```python
from build123d import *

# Parameters (mm, degrees)
SKETCH1_R                  = 15
BOSS_EXTRUDE1_DEPTH        = 210
FILLET1_R                  = 4
CHAMFER1_SIZE              = 1
M8X1_25_TAPPED_HOLE1_D     = 6.8
M8X1_25_TAPPED_HOLE1_DEPTH = 19.75
M8X1_25_TAPPED_HOLE1_TIP   = 2.042926105


with BuildPart() as part:
    # Sketch1 → Boss-Extrude1 (new body)
    with BuildSketch(Plane(origin=(0, 0, 0), x_dir=(1, 0, 0), z_dir=(0, 1, 0))):
        with Locations(Location((0, 0, 0), (0, 0, 270))):
            Circle(SKETCH1_R)
    extrude(amount=BOSS_EXTRUDE1_DEPTH)

    # Fillet1
    fillet1_edges = [part.edges().sort_by_distance(p)[0] for p in [
        (0, 0, -15),
    ]]
    fillet(fillet1_edges, radius=FILLET1_R)

    # Chamfer1
    chamfer1_edges = [part.edges().sort_by_distance(p)[0] for p in [
        (0, 210, -15),
    ]]
    chamfer(chamfer1_edges, length=CHAMFER1_SIZE)

    # M8x1.25 Tapped Hole1
    with Locations(Plane(origin=(0, 210, 0), x_dir=(1, 0, 0), z_dir=(0, 1, 0))):
        with Locations((0, 0)):
            Hole(M8X1_25_TAPPED_HOLE1_D / 2, depth=M8X1_25_TAPPED_HOLE1_DEPTH)
            with Locations((0, 0, -(M8X1_25_TAPPED_HOLE1_DEPTH + M8X1_25_TAPPED_HOLE1_TIP / 2))):  # 118° drill point
                Cone(0, M8X1_25_TAPPED_HOLE1_D / 2, M8X1_25_TAPPED_HOLE1_TIP, mode=Mode.SUBTRACT)


solid = part.part
```
The listing builds one solid part. Answer for the finished solid, in the listing's coordinates (mm). A direction names the side the tool comes from. Coordinates: 2 decimals unless noted, no trailing zeros. Write each loop counter-clockwise with the first axis right and the second up, starting at its lowest first coordinate (ties: lowest second). Pieces come first, ordered by that corner, then holes. Notation, with made-up numbers: M 33.25,35.25 L 43.25,35.25 A20 ccw 43.25,67.25 Z; hole C 66.5,34.5 d3. An arc over 180 degrees is marked long. Use a Markdown table: item, result. Add a question column.
1. Given P1, Ø6, axis at y = 36.5, z = 4, coming from the +X side; P2, Ø12, axis at x = 8.5, y = 27, coming from the -Z side; P3, Ø10, axis at y = 39.5, z = 10.5, coming from the +X side, each flat-ended and moving along its own axis, determine where each tip first touches the part or whether it passes through.
2. For a pull along Z with two mould halves and no side action, classify faces 1 (the conical face through (-0.128, 188.562, 0.576)), 2 (the cylindrical face through (0.66, 105.065, -14.985)), 3 (the flat face through (0, 0, 0)) as +Z half, -Z half, draft (parallel to the pull), parting line (faces both ways), or undercut.
3. Section B-B (y = 132.5) is taken. Give the vertices of the cut face in (x, z), plus the area to 3 significant figures.
4. Straight lines are drawn through the part: line 1 along Y through (x, z) = (-9.5, 6); line 2 along Z through (x, y) = (-3.5, 75.5); line 3 along Y through (x, z) = (-0.5, 3). For each, find the intervals that lie inside material, in ascending order. Write a range as [from, to].
5. Which of the six approach directions +Z, -Z, +X, -X, +Y, -Y give full straight-line access (tool end or side, diameter ignored) to faces 4 (the flat face through (-3, 210, 3)), 5 (the cylindrical face through (0.74, 199.99, 3.32))?
6. Section A-A (y = 194.5) is taken. Give the vertices of the cut face in (x, z), plus the area to 3 significant figures.
Data:
| question | item | result |
|---|---|---|
| 1 | P1 | stops at x = 14.97 |
| 1 | P2 | stops at z = -14.79 |
| 1 | P3 | stops at x = 13.96 |
| 2 | face 1 | undercut |
| 2 | face 2 | parting line |
| 2 | face 3 | draft |
| 3 | outline | C 0,0 d30 |
| 3 | area | 707 mm2 |
| 4 | line 1 | y = [0.01, 210] |
| 4 | line 2 | z = [-14.59, 14.59] |
| 4 | line 3 | y = [0, 190.03] |
| 5 | face 4 | +Z, -Z, +X, -X, +Y |
| 5 | face 5 | +Y |
| 6 | outline | C 0,0 d30; hole C 0,0 d6.8 |
| 6 | area | 671 mm2 |
